```python
from build123d import *

# Parameters (mm, degrees)
SKETCH1_R                = 121.5
BOSS_EXTRUDE1_DEPTH      = 10.09
BOSS_EXTRUDE2_DEPTH      = 10.11
BOSS_EXTRUDE2_DEPTH_BACK = 10.39
SKETCH2_R                = 24.795


with BuildPart() as part:
    # Sketch1 → Boss-Extrude1 (new, symmetric)
    with BuildSketch(Plane(origin=(0, 0, 0), x_dir=(1, 0, 0), z_dir=(0, 1, 0))):
        with Locations(Location((0, 0, 0), (0, 0, 270))):
            Circle(SKETCH1_R)
    extrude(amount=BOSS_EXTRUDE1_DEPTH, both=True)

    # Sketch2 → Boss-Extrude2 (add, two sides: drawn at the far end of the back side and taken through both)
    with BuildSketch(Plane(origin=(0, 0, 0), x_dir=(1, 0, 0), z_dir=(0, 1, 0)).offset(-BOSS_EXTRUDE2_DEPTH_BACK)):
        with Locations(Location((0, 0, 0), (0, 0, 270))):
            Circle(SKETCH2_R)
    extrude(amount=BOSS_EXTRUDE2_DEPTH + BOSS_EXTRUDE2_DEPTH_BACK)


solid = part.part
```
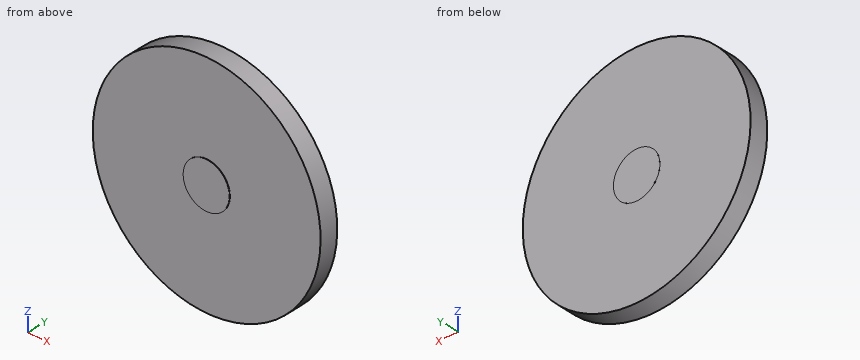
Can you work these out from the model? Positions are in its coordinate system, mm. Round coordinates to 2 decimals unless told otherwise and drop trailing zeros. Loops run counter-clockwise (first coordinate to the right, second up) from the corner with the lowest first, then second, coordinate; pieces in that order, holes last. Notation, with made-up numbers: M -16,62.5 L 9,62.5 A18 ccw 9,74.5 Z; hole C 41.25,29 d1. An arc over 180 degrees is marked long. Answer in a Markdown table with one row per item.
1. I'm going to push flat-ended pins straight in: pin 1 Ø1.5 at (y, z) = (-6.5, 7) entering from -X; pin 2 Ø1.5 at (x, y) = (-90.5, -5) entering from +Z; pin 3 Ø3 at (x, y) = (-16, 3.5) entering from +Z. Where does each tip first touch, or does it pass through?
Established:
| item | result |
|---|---|
| pin 1 | x = -121.34 |
| pin 2 | z = 81.9 |
| pin 3 | z = 120.63 |
2. Please list where these lines run through material, in increasing order: line 1 (Y direction, x = 39, z = 21); line 2 (X direction, y = -6.25, z = 11); line 3 (X direction, y = 2, z = -47.5). Write a range as from..to.
Established:
| item | result |
|---|---|
| line 1 | -10.09..10.09 |
| line 2 | -121..121 |
| line 3 | -111.83..111.83 |
3. If we section it at C-C, the plane x = 88.5: Please give me the cut outline in (y, z), plus the area to 3 significant figures.
Established:
| item | result |
|---|---|
| outline | M -10.09,-83.25 L 10.09,-83.25 L 10.09,83.25 L -10.09,83.25 Z |
| area | 3,360 mm² |
4. If we section it at D-D, the plane z = -50: Please give me the cut outline in (x, y).
Established:
| item | result |
|---|---|
| outline | M -110.74,-10.09 L 110.74,-10.09 L 110.74,10.09 L -110.74,10.09 Z |
5. If we section it at B-B, the plane y = 0: Please give me the cut outline in (x, z), plus the area to 3 significant figures.
Established:
| item | result |
|---|---|
| outline | C 0,0 d243 |
| area | 46,400 mm² |
